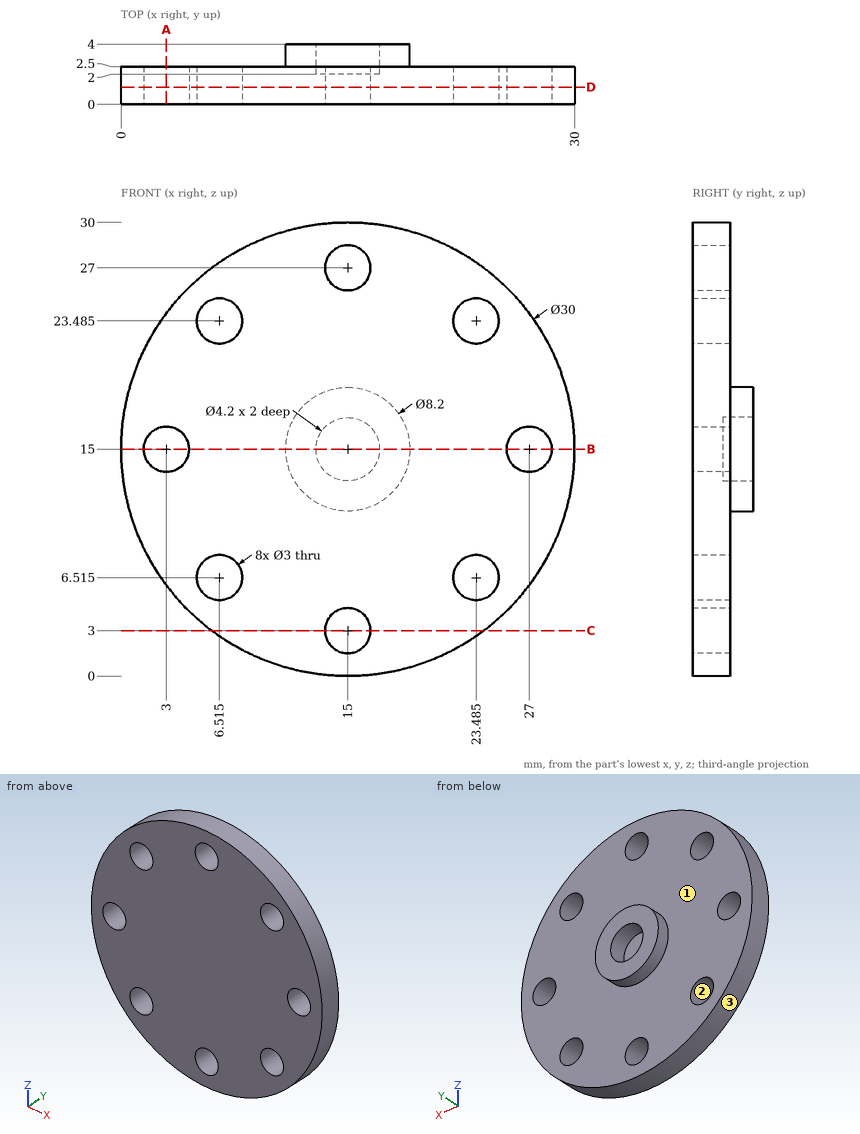
Geometry check sheet. Reference: drawing and pictorial views, mm from the part's lowest x, y, z. Round coordinates to 2 decimals unless told otherwise and drop trailing zeros. Loops run counter-clockwise (first coordinate to the right, second up) from the corner with the lowest first, then second, coordinate; pieces in that order, holes last. Notation, with made-up numbers: (76, 33.5) - (91, 33.5) arc R19 cw to (91, 48.5) - close; hole circle Ø9 at (48.5, 76). An arc over 180 degrees is marked (long way). Answer in a Markdown table with one row per item. Add a question column.
Q1. Gauge pin test, flat ends, axial feed: pin 1 (2.5 mm diameter, centred on x = 15, z = 27, fed in from -Y); pin 2 (1 mm diameter, centred on x = 9, y = 2.5, fed in from -Z) (1 decimal); pin 3 (1.5 mm diameter, centred on y = 2, z = 12, fed in from -X); pin 4 (1 mm diameter, centred on y = 0.5, z = 3, fed in from -X). Record the tip position at first contact, or that the pin passes through.
Q2. Section check A-A on x = 3. Enter the section's corners in (y, z), plus the area to 3 significant figures.
Q3. Section check D-D on y = 1.15. State how many separate pieces and enclosed holes the cut face has, plus the area to 3 significant figures.
Q4. Section check B-B on z = 15. Enter the section's corners in (x, y).
Q5. Section check C-C on z = 3. Enter the section's corners in (x, y), plus the area to 3 significant figures.
Q6. Material ranges on line 1 (X direction, y = 3.15, z = 15); line 2 (Y direction, x = 4.25, z = 13.75); line 3 (X direction, y = 2.15, z = 15.5) (1 decimal), recorded low to high.
Q7. Release check for a two-part mould opening along Z. For the marked faces 1, 2 and 3 record: pulls with the +Z half, pulls with the -Z half, needs draft (parallel to the pull), parting line crosses it, or undercut.
Found:
| question | item | result |
|---|---|---|
| 1 | pin 1 | passes through |
| 1 | pin 2 | stops at z = 1 |
| 1 | pin 3 | stops at x = 0.17 |
| 1 | pin 4 | stops at x = 5.37 |
| 2 | outline | (0, 6) - (2.5, 6) - (2.5, 13.5) - (0, 13.5) - close; (0, 16.5) - (2.5, 16.5) - (2.5, 24) - (0, 24) - close |
| 2 | area | 37.5 mm² |
| 3 | separate pieces | 1 |
| 3 | enclosed holes | 8 |
| 3 | area | 650 mm² |
| 4 | outline | (0, 0) - (1.5, 0) - (1.5, 2.5) - (0, 2.5) - close; (4.5, 0) - (25.5, 0) - (25.5, 2.5) - (19.1, 2.5) - (19.1, 4) - (17.1, 4) - (17.1, 2) - (12.9, 2) - (12.9, 4) - (10.9, 4) - (10.9, 2.5) - (4.5, 2.5) - close; (28.5, 0) - (30, 0) - (30, 2.5) - (28.5, 2.5) - close |
| 5 | outline | (6, 0) - (13.5, 0) - (13.5, 2.5) - (6, 2.5) - close; (16.5, 0) - (24, 0) - (24, 2.5) - (16.5, 2.5) - close |
| 5 | area | 37.5 mm² |
| 6 | line 1 | x = 10.9 to 12.9, 17.1 to 19.1 |
| 6 | line 2 | y = 0 to 2.5 |
| 6 | line 3 | x = 0 to 1.6, 4.4 to 13, 17 to 25.6, 28.4 to 30 |
| 7 | face 1 | needs draft |
| 7 | face 2 | undercut |
| 7 | face 3 | parting line crosses it |
